Geometry check sheet. Reference: the model listing, model coordinates, mm. A direction names the side the tool comes from. Round coordinates to 2 decimals unless told otherwise and drop trailing zeros. Write each loop counter-clockwise with the first axis right and the second up, starting at its lowest first coordinate (ties: lowest second). Pieces come first, ordered by that corner, then holes.
Item 1: Cross-section at D-D (y = -0.25). State how many separate pieces and enclosed holes the cut face has, then the cut area to 3 significant figures.
Item 2: Access from +Z, -Z, +X, -X, +Y, -Y to the whole of each face (thin tool, end or side, straight path). Record for faces 4 (the face through (1, -1, 1)), 5 (the face through (0.54, -2.44, 0.25)), 6 (the face through (-9, 0, 1)).
Item 3: Cross-section at A-A (x = 0). Enter the section's corners in (y, z).
Item 4: Cross-section at C-C (y = 1). Enter the section's corners in (x, z), then the cut area to 3 significant figures.
Item 5: Depth check by flat-ended pin: P1, Ø4, axis at x = 1, y = 0, coming from the -Z side; P2, Ø2.5, axis at x = -12, y = -0.5, coming from the +Z side; P3, Ø1, axis at y = 2.5, z = 3, coming from the -X side; P4, Ø4.5, axis at x = 0, y = 0, coming from the -Z side. Enter the tip coordinate at first touch or a pass-through.
Item 6: Cross-section at B-B (z = 4.65). Enter the section's corners in (x, y), then the cut area to 3 significant figures.
Item 7: Draft check along X on faces 1 (the face through (0.27, -1.22, 0.75)), 2 (the face through (-16, 0, 1)), 3 (the face through (-6, -1, 0)). Enter one of: pulls with the +X half, pulls with the -X half, needs draft (parallel to the pull), parting line crosses it, or undercut.
Item 8: Scan lines: probe 1 along Y at (x, z) = (0, 1.7); probe 2 along Z at (x, y) = (-7, 1.75); probe 3 along Y at (x, z) = (-1.5, 3.25). Record each from-to range of solid material in increasing order.
from build123d import *

# Parameters (mm, degrees)
EXTRUDE_3_DEPTH     = 2
EXTRUDE_3_2_DEPTH   = 2
SKETCH_2_R          = 3.75
SKETCH_2_R_2        = 2.5
EXTRUDE_5_DEPTH     = 3
SKETCH_3_R          = 3.75
SKETCH_3_R_2        = 2.5
EXTRUDE_6_DEPTH     = 2
SKETCH_4_R          = 0.5
CUT_EXTRUDE_1_DEPTH = 2
SKETCH_5_R          = 2.5
EXTRUDE_7_DEPTH     = 1
SKETCH_6_R          = 2.5
CUT_EXTRUDE_2_DEPTH = 0.5
SKETCH_7_R          = 1.25
CUT_EXTRUDE_3_DEPTH = 5
CUT_EXTRUDE1_DEPTH  = 6


with BuildPart() as part:
    # Sketch 1 → Extrude 3 (new body)
    with BuildSketch(Plane.XY):
        with BuildLine():
            ThreePointArc((-2.885471, -2.395111), (-3.527252, -1.273182), (-3.75, 0))
            ThreePointArc((-3.75, 0), (-3.527252, 1.273182), (-2.885471, 2.395111))
            Line((-2.885471, 2.395111), (-14.070828, 1.998745))
            ThreePointArc((-14.070828, 1.998745), (-16, 0), (-14.070828, -1.998745))
            Line((-14.070828, -1.998745), (-2.885471, -2.395111))
        make_face()
    extrude(amount=EXTRUDE_3_DEPTH)



with BuildPart() as body_2:
    # Sketch 1 → Extrude 3 2 (new body)
    with BuildSketch(Plane.XY):
        with BuildLine():
            Line((14.070828, 1.998745), (2.885471, 2.395111))
            ThreePointArc((2.885471, 2.395111), (3.75, 0), (2.885471, -2.395111))
            Line((2.885471, -2.395111), (14.070828, -1.998745))
            ThreePointArc((14.070828, -1.998745), (16, 0), (14.070828, 1.998745))
        make_face()
    extrude(amount=EXTRUDE_3_2_DEPTH)


with BuildPart() as body_3:
    # Sketch 2 → Extrude 5 (new body)
    with BuildSketch(Plane.XY.offset(2)):
        Circle(SKETCH_2_R)
        Circle(SKETCH_2_R_2, mode=Mode.SUBTRACT)
    extrude(amount=EXTRUDE_5_DEPTH)


with BuildPart() as part_1:
    add(part.part)

    add(body_2.part)  # Extrude 6 merges body 2

    add(body_3.part)  # Extrude 6 merges body 3
    # Sketch 3 → Extrude 6 (add)
    with BuildSketch(Plane(origin=(0, 0, 2), x_dir=(-1, 0, 0), z_dir=(0, 0, -1))):
        Circle(SKETCH_3_R)
        Circle(SKETCH_3_R_2, mode=Mode.SUBTRACT)
    extrude(amount=EXTRUDE_6_DEPTH)

    # Sketch 4 → Cut-Extrude 1 (cut)
    with BuildSketch(Plane(origin=(0, 0, 0), x_dir=(-1, 0, 0), z_dir=(0, 0, -1))):
        with Locations((-14.5, 0)):
            Circle(SKETCH_4_R)
        with Locations((-4.5, 0)):
            Circle(SKETCH_4_R)
        with Locations((-6.5, 0)):
            Circle(SKETCH_4_R)
        with Locations((-8.5, 0)):
            Circle(SKETCH_4_R)
        with Locations((-10.5, 0)):
            Circle(SKETCH_4_R)
        with Locations((-12.5, 0)):
            Circle(SKETCH_4_R)
        with Locations((4.5, 0)):
            Circle(SKETCH_4_R)
        with Locations((6.5, 0)):
            Circle(SKETCH_4_R)
        with Locations((8.5, 0)):
            Circle(SKETCH_4_R)
        with Locations((10.5, 0)):
            Circle(SKETCH_4_R)
        with Locations((12.5, 0)):
            Circle(SKETCH_4_R)
        with Locations((14.5, 0)):
            Circle(SKETCH_4_R)
    extrude(amount=-CUT_EXTRUDE_1_DEPTH, mode=Mode.SUBTRACT)

    # Sketch 5 → Extrude 7 (add)
    with BuildSketch(Plane(origin=(0, 0, 0), x_dir=(-1, 0, 0), z_dir=(0, 0, -1))):
        Circle(SKETCH_5_R)
    extrude(amount=-EXTRUDE_7_DEPTH)

    # Sketch 6 → Cut-Extrude 2 (cut)
    with BuildSketch(Plane(origin=(0, 0, 0), x_dir=(-1, 0, 0), z_dir=(0, 0, -1))):
        Circle(SKETCH_6_R)
    extrude(amount=-CUT_EXTRUDE_2_DEPTH, mode=Mode.SUBTRACT)

    # Sketch 7 → Cut-Extrude 3 (cut)
    with BuildSketch(Plane(origin=(0, 0, 0.5), x_dir=(-1, 0, 0), z_dir=(0, 0, -1))):
        Circle(SKETCH_7_R)
    extrude(amount=-CUT_EXTRUDE_3_DEPTH, mode=Mode.SUBTRACT)

    # Sketch1 → Cut-Extrude1 (cut, through all)
    with BuildSketch(Plane.XY.offset(5)):
        with BuildLine():
            ThreePointArc((3.75, 0), (3.527252, -1.273182), (2.885471, -2.395111))
            Line((2.885471, -2.395111), (14.070828, -1.998745))
            ThreePointArc((14.070828, -1.998745), (16, 0), (14.070828, 1.998745))
            Line((14.070828, 1.998745), (2.885471, 2.395111))
            ThreePointArc((2.885471, 2.395111), (3.527252, 1.273182), (3.75, 0))
        make_face()
    extrude(amount=-CUT_EXTRUDE1_DEPTH, mode=Mode.SUBTRACT)


solid = part_1.part
Resolved:
1. separate pieces: 8
1. enclosed holes: 0
1. area: 27.9 mm2
2. face 4: +Z
2. face 5: -Z
2. face 6: +Z, -Z
3. outline: (-3.75, 0) - (-2.5, 0) - (-2.5, 0.5) - (-1.25, 0.5) - (-1.25, 1) - (-2.5, 1) - (-2.5, 5) - (-3.75, 5) - close; (1.25, 0.5) - (2.5, 0.5) - (2.5, 0) - (3.75, 0) - (3.75, 5) - (2.5, 5) - (2.5, 1) - (1.25, 1) - close
4. outline: (-15.73, 0) - (-2.29, 0) - (-2.29, 0.5) - (-0.75, 0.5) - (-0.75, 1) - (-2.29, 1) - (-2.29, 5) - (-3.61, 5) - (-3.61, 2) - (-15.73, 2) - close; (0.75, 0.5) - (2.29, 0.5) - (2.29, 0) - (3.61, 0) - (3.61, 5) - (2.29, 5) - (2.29, 1) - (0.75, 1) - close
4. area: 39.0 mm2
5. P1: stops at z = 0
5. P2: stops at z = 2
5. P3: stops at x = -3.17
5. P4: stops at z = 0.5
6. outline: circle Ø7.5 at (0, 0); hole circle Ø5 at (0, 0)
6. area: 24.5 mm2
7. face 1: undercut
7. face 2: pulls with the -X half
7. face 3: needs draft
8. probe 1: y = -3.75 to -2.5, 2.5 to 3.75
8. probe 2: z = 0 to 2
8. probe 3: y = -3.44 to -2, 2 to 3.44
